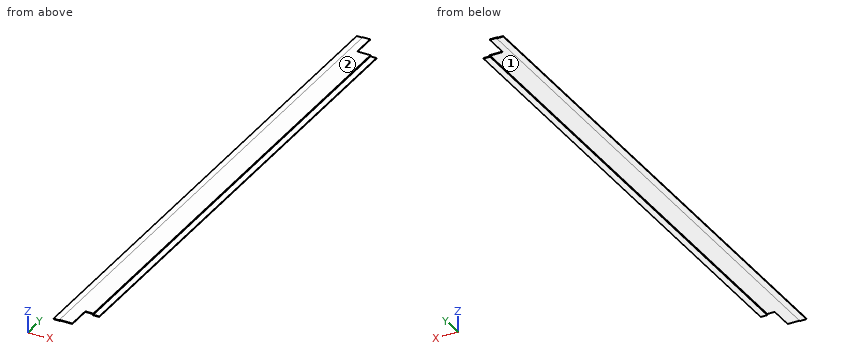
```python
from build123d import *

# Parameters (mm, degrees)
F1_DEPTH = 2312
F2_W     = 56.23
F2_H     = 99
F2_W_2   = 25
F2_W_3   = 33.5
F3_DEPTH = 7.501


# Not quite as in the source:
# - a feature names something its author has since deleted; it is built from what else it names


with BuildPart() as f1:
    # F0 (on Front) → F1 (new body)
    with BuildSketch(Plane.XZ):
        Polygon((87.5, 0), (0, 0), (0, -2), (-25, -2), (-25, -4.5), (2.5, -4.5), (2.5, -2.5), (85, -2.5), (85, -7.5), (112.5, -7.5), (112.5, -5), (87.5, -5), align=None)
    extrude(amount=F1_DEPTH)

    # F2 (on face) → F3 (cut, through all)
    with BuildSketch(Plane.XY):
        with Locations((59.385, -49.5)):
            Rectangle(F2_W, F2_H)
        with Locations((100, -49.5)):
            Rectangle(F2_W_2, F2_H)
        Polygon((127.1371338549, -2213), (87.5, -2213), (87.5, -2312), (54, -2312), (54, -2342.1576023102), (127.1371338549, -2342.1576023102), align=None)
        with Locations((70.75, -2262.5)):
            Rectangle(F2_W_3, F2_H)
    extrude(amount=-F3_DEPTH, mode=Mode.SUBTRACT)


solid = f1.part
```
Read the model definition and answer for the solid it produces. Units are mm, in the model's axes. Face numbers are marked on the shaded views. A direction names the side the tool comes from. Coordinates: 2 decimals unless noted, no trailing zeros. Write each loop counter-clockwise with the first axis right and the second up, starting at its lowest first coordinate (ties: lowest second). Pieces come first, ordered by that corner, then holes. Notation, with made-up numbers: (-12.75, 68) -> (16.25, 68) arc R5 cw to (16.25, 75) -> close; hole circle Ø11 at (39, 87). An arc over 180 degrees is marked (long way). Write item = value, one per line.
(1) Which of the six approach directions +Z, -Z, +X, -X, +Y, -Y give full straight-line access (tool end or side, diameter ignored) to the marked faces 1 and 2?
From the geometry:
face_1 = -Z, +Y, -Y
face_2 = +Z, +X, -X, +Y, -Y
(2) Section A-A on y = -239 is taken. Write down the section's boundary in (x, z), plus the area to 3 significant figures.
From the geometry:
outline = (-25, -4.5) -> (2.5, -4.5) -> (2.5, -2.5) -> (85, -2.5) -> (85, -7.5) -> (112.5, -7.5) -> (112.5, -5) -> (87.5, -5) -> (87.5, 0) -> (0, 0) -> (0, -2) -> (-25, -2) -> close
area = 361 mm2
(3) Given pin 1 Ø1.5 at (x, y) = (73.5, -764.5) entering from -Z; pin 2 Ø20 at (x, y) = (-11.5, -1567) entering from +Z; pin 3 Ø1 at (y, z) = (-988, -3.5) entering from +X, each flat-ended and moving along its own axis, determine where each tip first touches the part or whether it passes through.
From the geometry:
pin_1 = -2.5
pin_2 = -2
pin_3 = 87.5
(4) Straight lines are drawn through the part: L1, parallel to Z at x = 26.5, y = -409; L2, parallel to X at y = -1656, z = -5.75; L3, parallel to X at y = -589.5, z = -1. For each, find the intervals that lie inside material, in ascending order. Write a range as from..to.
From the geometry:
L1 = -2.5..0
L2 = 85..112.5
L3 = 0..87.5
